Could you check a few things on this model? Use its own coordinates, in mm. A direction names the side the tool comes from. Coordinates: 2 decimals unless noted, no trailing zeros. Write each loop counter-clockwise with the first axis right and the second up, starting at its lowest first coordinate (ties: lowest second). Pieces come first, ordered by that corner, then holes.
```python
from build123d import *

# Parameters (mm, degrees)
SCHIZZO1_W                   = 570
SCHIZZO1_H                   = 450
ESTRUSIONE_ESTRUSIONE1_DEPTH = 10
SCHIZZO2_R                   = 2.25
SCHIZZO2_W                   = 23
SCHIZZO2_H                   = 20
SCHIZZO2_W_2                 = 20
SCHIZZO2_H_2                 = 23
TAGLIO_ESTRUSIONE1_DEPTH     = 10
TAGLIO_ESTRUSIONE2_DEPTH     = 10


with BuildPart() as part:
    # Schizzo1 → Estrusione-Estrusione1 (new body)
    with BuildSketch(Plane(origin=(0, 0, 0), x_dir=(1, 0, 0), z_dir=(0, 1, 0))):
        with Locations((-285, 225)):
            Rectangle(SCHIZZO1_W, SCHIZZO1_H)
    extrude(amount=ESTRUSIONE_ESTRUSIONE1_DEPTH)

    # Schizzo2 → Taglio-Estrusione1 (cut)
    with BuildSketch(Plane.XZ):
        with Locations(Location((-467, -68, 0), (0, 0, 270))):
            Circle(SCHIZZO2_R)
        with Locations(Location((-448.5, -68, 0), (0, 0, 270))):
            Circle(SCHIZZO2_R)
        with Locations(Location((-121.5, -68, 0), (0, 0, 270))):
            Circle(SCHIZZO2_R)
        with Locations(Location((-103, -68, 0), (0, 0, 270))):
            Circle(SCHIZZO2_R)
        with Locations(Location((-467, -382, 0), (0, 0, 270))):
            Circle(SCHIZZO2_R)
        with Locations(Location((-448.5, -382, 0), (0, 0, 270))):
            Circle(SCHIZZO2_R)
        with Locations(Location((-121.5, -382, 0), (0, 0, 270))):
            Circle(SCHIZZO2_R)
        with Locations(Location((-103, -382, 0), (0, 0, 270))):
            Circle(SCHIZZO2_R)
        with Locations(Location((-472, -420, 0), (0, 0, 270))):
            Circle(SCHIZZO2_R)
        with Locations(Location((-540, -352, 0), (0, 0, 270))):
            Circle(SCHIZZO2_R)
        with Locations(Location((-540, -98, 0), (0, 0, 270))):
            Circle(SCHIZZO2_R)
        with Locations(Location((-472, -30, 0), (0, 0, 270))):
            Circle(SCHIZZO2_R)
        with Locations(Location((-98, -30, 0), (0, 0, 270))):
            Circle(SCHIZZO2_R)
        with Locations(Location((-30, -98, 0), (0, 0, 270))):
            Circle(SCHIZZO2_R)
        with Locations(Location((-30, -352, 0), (0, 0, 270))):
            Circle(SCHIZZO2_R)
        with Locations(Location((-98, -420, 0), (0, 0, 270))):
            Circle(SCHIZZO2_R)
        with Locations((-472, -10)):
            Rectangle(SCHIZZO2_W, SCHIZZO2_H)
        with Locations((-98, -10)):
            Rectangle(SCHIZZO2_W, SCHIZZO2_H)
        with Locations((-10, -98)):
            Rectangle(SCHIZZO2_W_2, SCHIZZO2_H_2)
        with Locations((-10, -352)):
            Rectangle(SCHIZZO2_W_2, SCHIZZO2_H_2)
        with Locations((-98, -440)):
            Rectangle(SCHIZZO2_W, SCHIZZO2_H)
        with Locations((-472, -440)):
            Rectangle(SCHIZZO2_W, SCHIZZO2_H)
        with Locations((-560, -352)):
            Rectangle(SCHIZZO2_W_2, SCHIZZO2_H_2)
        with Locations((-560, -98)):
            Rectangle(SCHIZZO2_W_2, SCHIZZO2_H_2)
    extrude(amount=-TAGLIO_ESTRUSIONE1_DEPTH, mode=Mode.SUBTRACT)

    # Schizzo3 → Taglio-Estrusione2 (cut)
    with BuildSketch(Plane.XZ):
        Polygon((-570, -225), (-551.2, -225), (-560.3, -215), (-522.7, -215), (-531.8, -225), (-513, -225), (-494.2, -225), (-503.3, -215), (-465.7, -215), (-474.8, -225), (-456, -225), (-437.2, -225), (-446.3, -215), (-408.7, -215), (-417.8, -225), (-399, -225), (-380.2, -225), (-389.3, -215), (-351.7, -215), (-360.8, -225), (-342, -225), (-323.2, -225), (-332.3, -215), (-294.7, -215), (-303.8, -225), (-285, -225), (-266.2, -225), (-275.3, -215), (-237.7, -215), (-246.8, -225), (-228, -225), (-209.2, -225), (-218.3, -215), (-180.7, -215), (-189.8, -225), (-171, -225), (-152.2, -225), (-161.3, -215), (-123.7, -215), (-132.8, -225), (-114, -225), (-95.2, -225), (-104.3, -215), (-66.7, -215), (-75.8, -225), (-57, -225), (-38.2, -225), (-47.3, -215), (-9.7, -215), (-18.8, -225), (0, -225), (0, -450), (-570, -450), align=None)
    extrude(amount=-TAGLIO_ESTRUSIONE2_DEPTH, mode=Mode.SUBTRACT)


solid = part.part
```
1. Please list where these lines run through material, in increasing order: line 1 along X through (y, z) = (3.5, -68); line 2 along Z through (x, y) = (-448.5, 3); line 3 along X through (y, z) = (3.25, -98).
Verdict:
line 1: x = -570 to -469.25, -464.75 to -450.75, -446.25 to -123.75, -119.25 to -105.25, -100.75 to 0
line 2: z = -225 to -70.25, -65.75 to 0
line 3: x = -550 to -542.25, -537.75 to -32.25, -27.75 to -20
2. If we mould it in two halves opening along Z, with no side actions, what happens to faces 1 (the face through (-114, 5, -225)), 2 (the face through (-98, 5, -20)), 3 (the face through (-470.186, 4.93, -219.93)), 4 (the face through (-527.186, 4.93, -219.93))? For each: pulls with the +Z half, pulls with the -Z half, needs draft (parallel to the pull), parting line crosses it, or undercut.
Verdict:
face 1: pulls with the -Z half
face 2: pulls with the +Z half
face 3: undercut
face 4: undercut
3. I want a section at A-A on y = 1.5. Give the number of separate pieces and of enclosed holes in the cut face, plus the area to 3 significant figures.
Verdict:
separate pieces: 1
enclosed holes: 8
area: 123,000 mm2
4. On a 3-axis mill with a long thin cutter (end or side, diameter ignored), from which of +Z, -Z, +X, -X, +Y, -Y can I reach the whole of each face in a straight line? I mean faces 5 (the face through (-20, 5, -98)), 6 (the face through (-57, 5, -225)), 7 (the face through (-29, 5, -215)), 8 (the face through (-560, 5, -86.5)). Say none if no direction works.
Verdict:
face 5: +X, +Y, -Y
face 6: -Z, +X, -X, +Y, -Y
face 7: +Y, -Y
face 8: -X, +Y, -Y
5. I want a section at B-B on x = -199. Please give me the cut outline in (y, z), plus the area to 3 significant figures.
Verdict:
outline: (0, -215) - (10, -215) - (10, 0) - (0, 0) - close
area: 2,150 mm2
6. For pin 1 (2.5 mm diameter, centred on x = -448.5, z = -68, fed in from +Y); pin 2 (3 mm diameter, centred on x = -27, y = 5.5, fed in from -Z); pin 3 (4 mm diameter, centred on y = 5, z = -105.5, fed in from -X), each with a flat end and sliding along its axis, tell me the tip position at first contact or that it passes through.
Verdict:
pin 1: passes through
pin 2: stops at z = -215
pin 3: stops at x = -550
